Source: CAD feature listing. Evaluate the final solid. Frame: model axes, mm. Face numbers are marked on the shaded views. Give positions to 0.01 mm unless a question says otherwise; leave off trailing zeros. Write each loop counter-clockwise with the first axis right and the second up, starting at its lowest first coordinate (ties: lowest second). Pieces come first, ordered by that corner, then holes. Notation, with made-up numbers: (79.25, -30.5) -> (128.25, -30.5) arc R32 ccw to (128.25, 5.5) -> close; hole circle Ø3 at (-39.75, 41). An arc over 180 degrees is marked (long way). Write item = value, one per line.
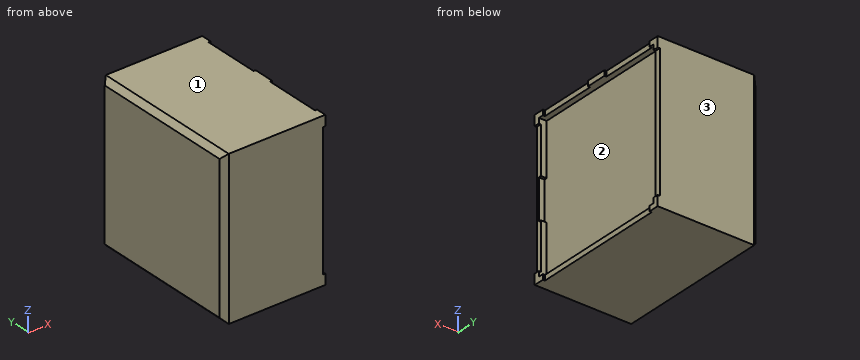
Autodesk Inventor part; units mm, degrees
ref_plane "body_to_dummy_sk_XY" through (-11.4046, 0, 0) normal (-1, 0, 0) x (0, 0, -1)
ref_plane "body_to_dummy_sk_YZ" through (-11.4046, 0, 0) normal (0, 0, -1) x (0, -1, 0)
ref_plane "body_to_dummy_sk_ZX" through (-11.4046, 0, 0) normal (0, -1, 0) x (-1, 0, 0)
sketch "Sketch_2" plane through (1.016, 0, 0) normal (1, 0, 0) x (0, 0, -1)
  line L0 (-7.62, -7.62) -> (7.62, -7.62)
  line L1 (7.62, -7.62) -> (7.62, 7.62)
  line L2 (7.62, 7.62) -> (-7.62, 7.62)
  line L3 (-7.62, 7.62) -> (-7.62, -7.62)
extrude "Extrusion1" add sketch "Sketch_2" against normal blind 10.0076
sketch "Sketch_1" plane through (1.016, 0, 0) normal (1, 0, 0) x (0, 0, -1)
  line L0 (-7.112, -7.112) -> (-1.9812, -7.112)
  line L1 (-1.9812, -7.112) -> (-1.9812, -7.366)
  line L2 (-1.9812, -7.366) -> (1.9812, -7.366)
  line L3 (1.9812, -7.366) -> (1.9812, -7.112)
  line L4 (1.9812, -7.112) -> (7.112, -7.112)
  line L5 (7.112, -7.112) -> (7.112, 7.112)
  line L6 (7.112, 7.112) -> (-7.112, 7.112)
  line L7 (-7.112, 7.112) -> (-7.112, -7.112)
extrude "Extrusion2" cut sketch "Sketch_1" against normal blind 0.762
sketch "Sketch_3" plane through (0, 0, 0) normal (0, 0, 1) x (1, 0, 0)
  line L0 (-18.9992, 7.62) -> (-18.9992, -7.62)
  line L1 (-18.9992, -7.62) -> (-8.4836, -7.62)
  line L2 (-8.4836, -7.62) -> (-8.9916, -7.112)
  line L3 (-8.9916, -7.112) -> (-8.9916, 7.112)
  line L4 (-8.9916, 7.112) -> (-8.4836, 7.62)
  line L5 (-8.4836, 7.62) -> (-18.9992, 7.62)
extrude "Extrusion3" cut sketch "Sketch_3" along normal mid plane 15.24
sketch "Sketch_4" plane through (0, 0, 0) normal (0, 1, 0) x (-1, 0, 0)
  line L0 (18.9992, -7.62) -> (18.9992, 7.62)
  line L1 (18.9992, 7.62) -> (8.4836, 7.62)
  line L2 (8.4836, 7.62) -> (8.9916, 7.112)
  line L3 (8.9916, 7.112) -> (8.9916, -7.112)
  line L4 (8.9916, -7.112) -> (8.4836, -7.62)
  line L5 (8.4836, -7.62) -> (18.9992, -7.62)
extrude "Extrusion4" cut sketch "Sketch_4" along normal mid plane 15.24
sketch "Sketch_5" plane through (0, 7.62, 0) normal (0, 1, 0) x (1, 0, 0)
  line L0 (0.8128, 6.604) -> (0.8128, -6.604)
  line L1 (0.8128, -6.604) -> (1.016, -6.604)
  line L2 (1.016, -6.604) -> (1.016, 6.604)
  line L3 (1.016, 6.604) -> (0.8128, 6.604)
extrude "Extrusion5" cut sketch "Sketch_5" against normal blind 15.24
sketch "Sketch_6" plane through (0, 0, -7.62) normal (0, 0, 1) x (1, 0, 0)
  line L0 (0.8128, 6.604) -> (0.8128, -6.604)
  line L1 (0.8128, -6.604) -> (1.016, -6.604)
  line L2 (1.016, -6.604) -> (1.016, 6.604)
  line L3 (1.016, 6.604) -> (0.8128, 6.604)
extrude "Extrusion6" cut sketch "Sketch_6" along normal blind 0.508
sketch "Sketch_7" plane through (0, 0, 7.62) normal (0, 0, 1) x (1, 0, 0)
  line L0 (0.8128, 6.604) -> (0.8128, 1.016)
  line L1 (0.8128, 1.016) -> (1.016, 1.016)
  line L2 (1.016, 1.016) -> (1.016, 6.604)
  line L3 (1.016, 6.604) -> (0.8128, 6.604)
extrude "Extrusion7" cut sketch "Sketch_7" against normal blind 0.508
sketch "Sketch_8" plane through (0, 0, 7.62) normal (0, 0, 1) x (1, 0, 0)
  line L0 (0.8128, -1.016) -> (0.8128, -6.604)
  line L1 (0.8128, -6.604) -> (1.016, -6.604)
  line L2 (1.016, -6.604) -> (1.016, -1.016)
  line L3 (1.016, -1.016) -> (0.8128, -1.016)
extrude "Extrusion8" cut sketch "Sketch_8" against normal blind 0.508
ref_plane "body_to_dummy_sk_XY" through (-11.4046, 0, 0) normal (-1, 0, 0) x (0, 0, -1)
ref_plane "body_to_dummy_sk_YZ" through (-11.4046, 0, 0) normal (0, 0, -1) x (0, -1, 0)
ref_plane "body_to_dummy_sk_ZX" through (-11.4046, 0, 0) normal (0, -1, 0) x (-1, 0, 0)
ref_plane "body_to_dummy_sk_green_XY" through (-11.4046, 0, -3.7529) normal (-1, 0, 0) x (0, 0, -1)
ref_plane "body_to_dummy_sk_green_YZ" through (-11.4046, 0, -3.7529) normal (0, 0, -1) x (0, -1, 0)
ref_plane "body_to_dummy_sk_green_ZX" through (-11.4046, 0, -3.7529) normal (0, -1, 0) x (-1, 0, 0)
ref_plane "body_to_dummy_sk_red_XY" through (-11.4046, 0, 3.7529) normal (-1, 0, 0) x (0, 0, -1)
ref_plane "body_to_dummy_sk_red_YZ" through (-11.4046, 0, 3.7529) normal (0, 0, -1) x (0, -1, 0)
ref_plane "body_to_dummy_sk_red_ZX" through (-11.4046, 0, 3.7529) normal (0, -1, 0) x (-1, 0, 0)
ref_plane "body_to_pole_XY" through (-0.508, 0, 0) normal (-1, 0, 0) x (0, 0, -1)
ref_plane "body_to_pole_YZ" through (-0.508, 0, 0) normal (0, 0, -1) x (0, -1, 0)
ref_plane "body_to_pole_ZX" through (-0.508, 0, 0) normal (0, -1, 0) x (-1, 0, 0)
properties part number "UB21SK035D-1JBbody"
(1) Section query A-A (z = 1.5). Return loops of the section in (x, y).
Values follow:
outline = (-8.99, -7.11) -> (-8.48, -7.62) -> (0.81, -7.62) -> (0.81, -7.37) -> (0.25, -7.37) -> (0.25, 7.11) -> (0.81, 7.11) -> (0.81, 7.62) -> (-8.48, 7.62) -> (-8.99, 7.11) -> close
(2) Section query B-B (y = -0.25). Return loops of the section in (x, z), plus the area to 3 significant figures.
Values follow:
outline = (-8.99, -7.11) -> (-8.48, -7.62) -> (0.81, -7.62) -> (0.81, -7.11) -> (0.25, -7.11) -> (0.25, 7.11) -> (1.02, 7.11) -> (1.02, 7.62) -> (-8.48, 7.62) -> (-8.99, 7.11) -> close
area = 141 mm2
(3) Pull-direction query (Z, two-part tool) for the marked faces 1, 2 and 3; classes: pulls with the +Z half, pulls with the -Z half, needs draft (parallel to the pull), parting line crosses it, or undercut.
Values follow:
face_1 = pulls with the +Z half
face_2 = undercut
face_3 = needs draft
(4) First-contact query: pin 1 (4.5 mm diameter, centred on y = 1.5, z = 1, fed in from +X); pin 2 (0.6 mm diameter, centred on y = 7.5, z = 2, fed in from +X). Flat tips, straight axial feed; report the tip coordinate or a pass-through.
Values follow:
pin_1 = 0.25
pin_2 = 0.81
(5) Material intervals for line 1 (X direction, y = 5.75, z = 1), sorted ascending.
Values follow:
line_1 = -8.99 to 0.25
